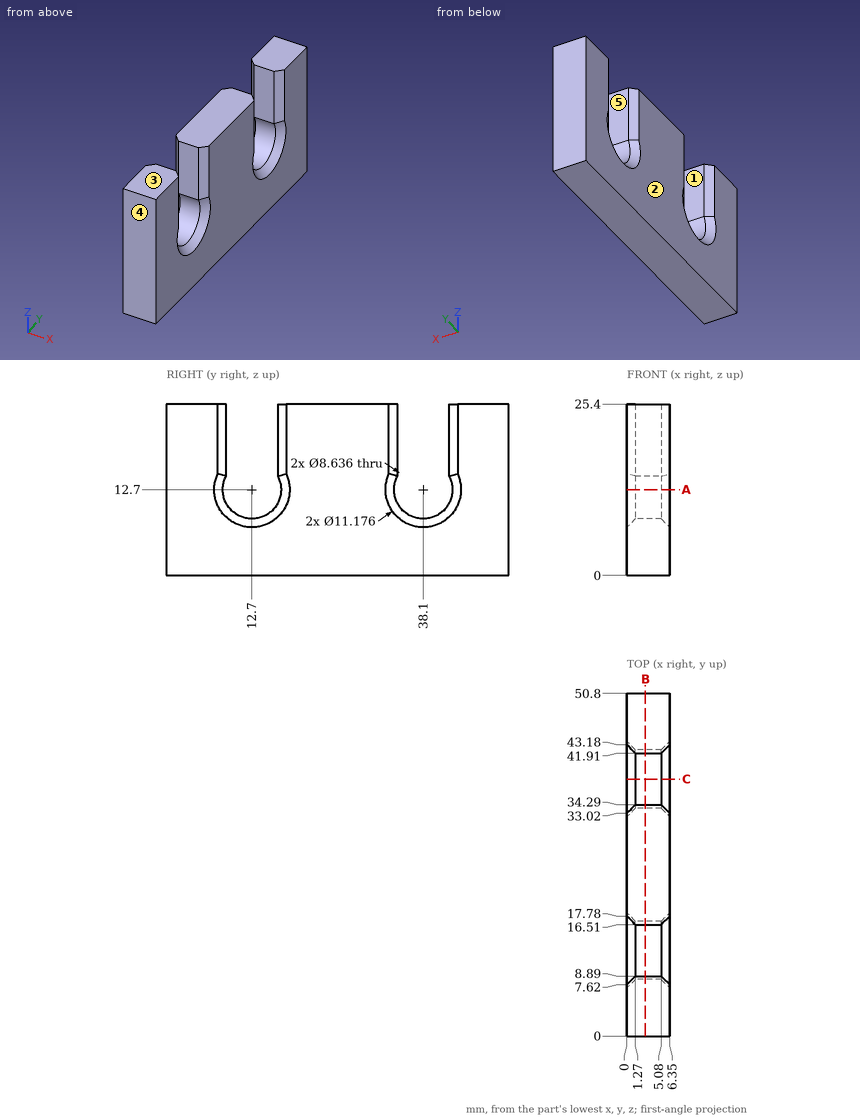
Check sheet for the drawn part. Datum: minimum x, y, z corner. Units: mm. A direction names the side the tool comes from. Coordinates: 2 decimals unless noted, no trailing zeros. Order: outer loops, then holes, each group sorted by start corner. A loop starts at its lowest first (then second) coordinate and runs counter-clockwise, first axis right, second up. Notation, with made-up numbers: (75.5, 65) -> (123.5, 65) arc R31 cw to (123.5, 100) -> close; hole circle Ø3 at (75, 8.5). An arc over 180 degrees is marked (long way). Write each question's results on one line, items separated by ' | '. Start each with the question number.
1) Set-up check for the marked faces 1 and 2: record each of +Z, -Z, +X, -X, +Y, -Y from which the full face is reachable in a straight line by a thin tool's end or side.
2) Section check B-B (x = 2.75). Enter the section's corners in (y, z), and give its area (3 significant figures).
3) Draft check along Y on the marked faces 3, 4 and 5. Enter one of: pulls with the +Y half, pulls with the -Y half, needs draft (parallel to the pull), parting line crosses it, or undercut.
4) Material ranges on line 1 along Y through (x, z) = (3.1, 12.7); line 2 along Y through (x, z) = (5, 19.75); line 3 along Z through (x, y) = (3, 12.7), recorded low to high.
5) Depth check by flat-ended pin: pin 1 (6 mm diameter, centred on y = 40, z = 14, fed in from -X). Enter the tip coordinate at first touch or a pass-through.
6) Section check A-A (z = 12.7). Enter the section's corners in (x, y), and give its area (3 significant figures).
7) Section check C-C (y = 38.1). Enter the section's corners in (x, z), and give its area (3 significant figures).
Checked values:
1) face 1: +Z, +X, -X | face 2: +Z, -Z, -X, +Y, -Y
2) outline: (0, 0) -> (50.8, 0) -> (50.8, 25.4) -> (41.91, 25.4) -> (41.91, 14.73) arc R4.32 cw (long way) to (34.29, 14.73) -> (34.29, 25.4) -> (16.51, 25.4) -> (16.51, 14.73) arc R4.32 cw (long way) to (8.89, 14.73) -> (8.89, 25.4) -> (0, 25.4) -> close | area: 1,040 mm²
3) face 3: needs draft | face 4: pulls with the -Y half | face 5: undercut
4) line 1: 0 to 8.38, 17.02 to 33.78, 42.42 to 50.8 | line 2: 0 to 8.89, 16.51 to 34.29, 41.91 to 50.8 | line 3: 0 to 8.38
5) pin 1: x = 0.34
6) outline: (0, 0) -> (6.35, 0) -> (6.35, 7.11) -> (5.08, 8.38) -> (1.27, 8.38) -> (0, 7.11) -> close; (0, 18.29) -> (1.27, 17.02) -> (5.08, 17.02) -> (6.35, 18.29) -> (6.35, 32.51) -> (5.08, 33.78) -> (1.27, 33.78) -> (0, 32.51) -> close; (0, 43.69) -> (1.27, 42.42) -> (5.08, 42.42) -> (6.35, 43.69) -> (6.35, 50.8) -> (0, 50.8) -> close | area: 206 mm²
7) outline: (0, 0) -> (6.35, 0) -> (6.35, 7.11) -> (5.08, 8.38) -> (1.27, 8.38) -> (0, 7.11) -> close | area: 51.6 mm²
